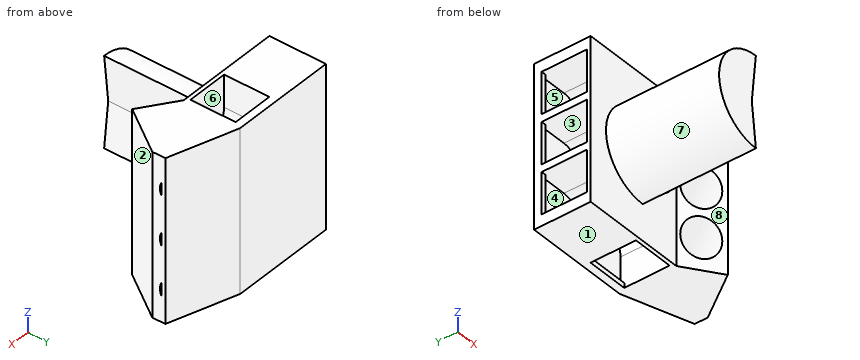
from build123d import *

# Parameters (mm, degrees)
HOUSING_DEPTH                  = 3
KINK_HOUSING_DEPTH             = 8.6
KINK_SLOTS_REACH               = 11.941
KINK_SLOTS_OFFSET_FROM_SURFACE = 0.2
SKETCH18_RX                    = 1.1
SKETCH18_RY                    = 0.901067249
SIDE_START                     = 0.2
SKETCH1_14_R                   = 1.1
SIDE_CUTS_DEPTH                = 2.6
SKETCH1_15_R                   = 1.1
CENTER_CUT_DEPTH               = 2.8
BOSS_EXTRUDE4_START            = -0.2
BOSS_EXTRUDE4_DEPTH            = 0.2
BOSS_EXTRUDE5_DEPTH            = 6


with BuildPart() as part:
    # Sketch1 → Housing (new body)
    with BuildSketch(Plane(origin=(0, 0, 0), x_dir=(1, 0, 0), z_dir=(0, 1, 0))):
        Polygon((3.9, 6.9), (-1.7, 6.9), (-1.7, -1.7), (3.9, -1.7), (3.9, 5.2), align=None)
    extrude(amount=HOUSING_DEPTH)

    # Sketch1<14> → Side Cuts (cut)
    with BuildSketch(Plane(origin=(0, 0, 0), x_dir=(1, 0, 0), z_dir=(0, 1, 0)).offset(SIDE_START)):
        with BuildLine():
            Line((3.7, 5.2), (3.7, 6.9))
            Line((3.7, 6.9), (1.5, 6.9))
            Line((1.5, 6.9), (1.5, 5.2))
            ThreePointArc((1.5, 5.2), (2.6, 6.3), (3.7, 5.2))
        make_face()
        with Locations((2.6, 5.2)):
            Circle(SKETCH1_14_R)
        with Locations((0, 5.2)):
            Circle(SKETCH1_14_R)
        with BuildLine():
            Line((0, 6.3), (-1.7, 6.3))
            Line((-1.7, 6.3), (-1.7, 4.1))
            Line((-1.7, 4.1), (0, 4.1))
            ThreePointArc((0, 4.1), (-1.1, 5.2), (0, 6.3))
        make_face()
        with Locations((0, 2.6)):
            Circle(SKETCH1_14_R)
        with BuildLine():
            Line((0, 3.7), (-1.7, 3.7))
            Line((-1.7, 3.7), (-1.7, 1.5))
            Line((-1.7, 1.5), (0, 1.5))
            ThreePointArc((0, 1.5), (-1.1, 2.6), (0, 3.7))
        make_face()
        with Locations((2.6, 0)):
            Circle(SKETCH1_14_R)
        with BuildLine():
            Line((1.5, -1.7), (3.7, -1.7))
            Line((3.7, -1.7), (3.7, 0))
            ThreePointArc((3.7, 0), (2.6, -1.1), (1.5, 0))
            Line((1.5, 0), (1.5, -1.7))
        make_face()
        Circle(SKETCH1_14_R)
        with BuildLine():
            Line((-1.7, 1.1), (-1.7, -1.1))
            Line((-1.7, -1.1), (0, -1.1))
            ThreePointArc((0, -1.1), (-1.1, 0), (0, 1.1))
            Line((0, 1.1), (-1.7, 1.1))
        make_face()
    extrude(amount=SIDE_CUTS_DEPTH, mode=Mode.SUBTRACT)

    # Sketch1<15> → Center Cut (cut)
    with BuildSketch(Plane(origin=(0, 0, 0), x_dir=(1, 0, 0), z_dir=(0, 1, 0))):
        with Locations(Location((2.6, 2.6, 0), (0, 0, 270))):
            Circle(SKETCH1_15_R)
    extrude(amount=CENTER_CUT_DEPTH, mode=Mode.SUBTRACT)



with BuildPart() as body_2:
    # Tilted Magnet → Kink Housing (new body)
    with BuildSketch(Plane(origin=(0, 0, -6.9), x_dir=(-1, 0, 0), z_dir=(0, 0, -1))):
        Polygon((-3.9, 3), (-7.422863806, 1.889245308), (-7.422863806, 1.195587973), (-5.702134497, -1.26186816), (-3.9, 0), align=None)
    extrude(amount=-KINK_HOUSING_DEPTH)

    # Kink Slots: up to this face of the body (flat: up to its plane, moved by the offset)
    kink_slots_end = Plane(body_2.part.faces().sort_by_distance((5.661431903, 2.444622654, -2.6))[0]).offset(-KINK_SLOTS_OFFSET_FROM_SURFACE)
    # Sketch18 → Kink Slots (cut, up to the picked face)
    with BuildSketch(Plane(origin=(1.283060721, 1.832400611, 0), x_dir=(0.8191520442889985, -0.5735764363510366, 0), z_dir=(-0.5735764363510366, -0.8191520442889985, 0)), mode=Mode.PRIVATE) as kink_slots_sk1:
        with Locations(Location((4.25959063, -5.2), (0, 0, 90))):
            Ellipse(SKETCH18_RX, SKETCH18_RY)
    kink_slots_tool1 = split(extrude(kink_slots_sk1.sketch, amount=-KINK_SLOTS_REACH, mode=Mode.PRIVATE), bisect_by=kink_slots_end, keep=Keep.BOTH, mode=Mode.PRIVATE)
    # Sketch18 → Kink Slots (cut, up to the picked face)
    with BuildSketch(Plane(origin=(1.283060721, 1.832400611, 0), x_dir=(0.8191520442889985, -0.5735764363510366, 0), z_dir=(-0.5735764363510366, -0.8191520442889985, 0)), mode=Mode.PRIVATE) as kink_slots_sk2:
        with Locations(Location((4.25959063, -2.6), (0, 0, -90))):
            Ellipse(SKETCH18_RX, SKETCH18_RY)
    kink_slots_tool2 = split(extrude(kink_slots_sk2.sketch, amount=-KINK_SLOTS_REACH, mode=Mode.PRIVATE), bisect_by=kink_slots_end, keep=Keep.BOTH, mode=Mode.PRIVATE)
    # Sketch18 → Kink Slots (cut, up to the picked face)
    with BuildSketch(Plane(origin=(1.283060721, 1.832400611, 0), x_dir=(0.8191520442889985, -0.5735764363510366, 0), z_dir=(-0.5735764363510366, -0.8191520442889985, 0)), mode=Mode.PRIVATE) as kink_slots_sk3:
        with Locations(Location((4.25959063, 0), (0, 0, 90))):
            Ellipse(SKETCH18_RX, SKETCH18_RY)
    kink_slots_tool3 = split(extrude(kink_slots_sk3.sketch, amount=-KINK_SLOTS_REACH, mode=Mode.PRIVATE), bisect_by=kink_slots_end, keep=Keep.BOTH, mode=Mode.PRIVATE)
    add(kink_slots_tool1.solids().sort_by(Axis((4.772313, -0.6108, -5.2), (0.5735764363510366, 0.8191520442889985, 0)))[0], mode=Mode.SUBTRACT)
    add(kink_slots_tool2.solids().sort_by(Axis((4.772313, -0.6108, -2.6), (0.5735764363510366, 0.8191520442889985, 0)))[0], mode=Mode.SUBTRACT)
    add(kink_slots_tool3.solids().sort_by(Axis((4.772313, -0.6108, 0), (0.5735764363510366, 0.8191520442889985, 0)))[0], mode=Mode.SUBTRACT)


with BuildPart() as part_1:
    add(part.part)

    add(body_2.part)  # Boss-Extrude4 merges body 2
    # Sketch19 → Boss-Extrude4 (add)
    with BuildSketch(Plane(origin=(0, 3, 0), x_dir=(1, 0, 0), z_dir=(0, 1, 0)).offset(BOSS_EXTRUDE4_START)):
        Polygon((3.9, 6.9), (-1.7, 6.9), (-1.7, -1.7), (3.9, -1.7), (3.9, -1.440815164), (-1.440815164, -1.440815164), (-1.440815164, 6.640815164), (3.9, 6.640815164), align=None)
    extrude(amount=-BOSS_EXTRUDE4_DEPTH)

    # Sketch20 → Boss-Extrude5 (add)
    with BuildSketch(Plane.XZ):
        with BuildLine():
            Line((1.432886326, -2.7), (1.7, -0.2))
            ThreePointArc((1.7, -0.2), (-0.7, -2.6), (1.7, -5))
            Line((1.7, -5), (1.432886326, -2.7))
        make_face()
    extrude(amount=BOSS_EXTRUDE5_DEPTH)


solid = part_1.part
Work out the finished part from the listing and answer in its coordinate system (mm). Face numbers are marked on the shaded views. A direction names the side the tool comes from. Give positions to 0.01 mm unless a question says otherwise; leave off trailing zeros. Order: outer loops, then holes, each group sorted by start corner. A loop starts at its lowest first (then second) coordinate and runs counter-clockwise, first axis right, second up. Notation, with made-up numbers: (74, 16) - (118, 16) arc R26 cw to (118, 35) - close; hole circle Ø2 at (-13, 78). An arc over 180 degrees is marked (long way). Answer as CSV lines item,"result". Start each with the question number.
Q1. The mould has two halves that part along Y. Classify the marked faces 1, 2, 3 and 4: +Y half, -Y half, draft (parallel to the pull), parting line (faces both ways), or undercut.
Q2. Given pin 1 Ø1 at (y, z) = (-0.5, -4) entering from +X; pin 2 Ø2 at (x, z) = (5, -6) entering from -Y; pin 3 Ø1.9 at (y, z) = (1, 1) entering from +X; pin 4 Ø4 at (x, y) = (4.5, -3) entering from +Z, each flat-ended and moving along its own axis, determine where each tip first touches the part or whether it passes through.
Q3. The part is cut by section B-B (x = 0.25). Write down the section's boundary in (y, z), then the cut area to 3 significant figures.
Q4. Find the intervals of material crossed by L1, parallel to Z at x = -0.5, y = 2.5; L2, parallel to Y at x = 3.5, z = -5; L3, parallel to X at y = 1.25, z = -2.6, in increasing order. Write a range as [from, to].
Q5. The part is cut by section C-C (y = -4). Write down the section's boundary in (x, z), then the cut area to 3 significant figures.
Q6. For the marked faces 5, 6, 7 and 8, determine the directions among +Z, -Z, +X, -X, +Y, -Y from which every point of the face is accessible in a straight line to the end or side of a thin tool.
Q7. The part is cut by section A-A (x = 2.6). Write down the section's boundary in (y, z).
Check result:
1,face 1,"draft"
1,face 2,"-Y half"
1,face 3,"undercut"
1,face 4,"undercut"
2,pin 1,"stops at x = 6.59"
2,pin 2,"stops at y = -1.26"
2,pin 3,"stops at x = 7.42"
2,pin 4,"passes through"
3,outline,"(-6, -4.51) - (0, -4.51) - (0, -6.9) - (3, -6.9) - (3, 1.7) - (0, 1.7) - (0, -0.69) - (-6, -0.69) - close; hole (0.2, -6.27) - (2.8, -6.27) - (2.8, -4.13) - (0.2, -4.13) - close; hole (0.2, -3.67) - (2.8, -3.67) - (2.8, -1.53) - (0.2, -1.53) - close; hole (0.2, -1.07) - (2.8, -1.07) - (2.8, 1.07) - (0.2, 1.07) - close"
3,area,"32.0 mm²"
4,L1,"z = [-6.9, -6.3], [-4.1, -3.7], [-1.5, -1.1], [1.1, 1.7]"
4,L2,"y = [0, 0.2], [2.8, 3]"
4,L3,"x = [1.1, 1.5], [3.7, 4.98], [7.18, 7.42]"
5,outline,"(1.43, -2.7) - (1.7, -0.2) arc R2.4 ccw to (1.7, -5) - close"
5,area,"8.41 mm²"
6,face 5,"none"
6,face 6,"+Z"
6,face 7,"-X, -Y"
6,face 8,"+Z, -Z, -Y"
7,outline,"(0, -6.9) - (0.2, -6.9) - (0.2, -4.1) - (2.8, -4.1) - (2.8, -6.64) - (2.6, -6.64) - (2.6, -6.9) - (3, -6.9) - (3, 1.7) - (2.6, 1.7) - (2.6, 1.44) - (2.8, 1.44) - (2.8, -1.1) - (0.2, -1.1) - (0.2, 1.7) - (0, 1.7) - (0, -1.5) - (2.8, -1.5) - (2.8, -3.7) - (0, -3.7) - close"
